```python
from build123d import *

# Parameters (mm, degrees)
SKETCH1_R                = 5
SKETCH1_R_2              = 4
BOSS_EXTRUDE1_DEPTH      = 5
BOSS_EXTRUDE3_DEPTH      = 7.5
BOSS_EXTRUDE3_DEPTH_BACK = 12.5
SKETCH2_R                = 7
SKETCH2_R_2              = 5
SKETCH3_R                = 5
BOSS_EXTRUDE4_DEPTH      = 5
FILLET1_R                = 4


with BuildPart() as part:
    # Sketch1 → Boss-Extrude1 (new body)
    with BuildSketch(Plane(origin=(0, 0, 0), x_dir=(0, 0, -1), z_dir=(1, 0, 0))):
        with BuildLine():
            Line((50, 221.0514346), (50, 161.0514346))
            ThreePointArc((50, 161.0514346), (26.21791649, 82.161607759), (20, 0))
            ThreePointArc((20, 0), (0, -20), (-20, 0))
            ThreePointArc((-20, 0), (-3.28398519, 116.315677296), (50, 221.0514346))
        make_face()
        Circle(SKETCH1_R, mode=Mode.SUBTRACT)
        with Locations((0, 47.625)):
            Circle(SKETCH1_R_2, mode=Mode.SUBTRACT)
        with Locations((1.573444046, 62.542247529)):
            Circle(SKETCH1_R_2, mode=Mode.SUBTRACT)
        with Locations((3.912796623, 77.358705591)):
            Circle(SKETCH1_R_2, mode=Mode.SUBTRACT)
        with Locations((7.013151247, 92.034801844)):
            Circle(SKETCH1_R_2, mode=Mode.SUBTRACT)
        with Locations((10.86160852, 106.532711232)):
            Circle(SKETCH1_R_2, mode=Mode.SUBTRACT)
        with Locations((15.437856468, 120.817596765)):
            Circle(SKETCH1_R_2, mode=Mode.SUBTRACT)
        with Locations((20.715135496, 134.858619736)):
            Circle(SKETCH1_R_2, mode=Mode.SUBTRACT)
        with Locations((26.661473463, 148.629642385)):
            Circle(SKETCH1_R_2, mode=Mode.SUBTRACT)
        with Locations((33.241055411, 162.109594216)):
            Circle(SKETCH1_R_2, mode=Mode.SUBTRACT)
        with Locations((-0.810748538, 32.646926465)):
            Circle(SKETCH1_R_2, mode=Mode.SUBTRACT)
    extrude(amount=BOSS_EXTRUDE1_DEPTH)

    # Sketch2 → Boss-Extrude3 (add, two sides: drawn at the far end of the back side and taken through both)
    with BuildSketch(Plane(origin=(5, 0, 0), x_dir=(0, 0, -1), z_dir=(1, 0, 0)).offset(-BOSS_EXTRUDE3_DEPTH_BACK)):
        Circle(SKETCH2_R)
        Circle(SKETCH2_R_2, mode=Mode.SUBTRACT)
    extrude(amount=BOSS_EXTRUDE3_DEPTH + BOSS_EXTRUDE3_DEPTH_BACK)

    # Sketch3 → Boss-Extrude4 (add)
    with BuildSketch(Plane(origin=(0, 0, -50), x_dir=(-1, 0, 0), z_dir=(0, 0, -1))):
        with BuildLine():
            Line((-12.5, 151.0514346), (7.5, 151.0514346))
            ThreePointArc((7.5, 151.0514346), (14.571067812, 153.980366789), (17.5, 161.0514346))
            Line((17.5, 161.0514346), (17.5, 221.0514346))
            ThreePointArc((17.5, 221.0514346), (14.571067812, 228.122502412), (7.5, 231.0514346))
            Line((7.5, 231.0514346), (-12.5, 231.0514346))
            ThreePointArc((-12.5, 231.0514346), (-19.571067812, 228.122502412), (-22.5, 221.0514346))
            Line((-22.5, 221.0514346), (-22.5, 161.0514346))
            ThreePointArc((-22.5, 161.0514346), (-19.571067812, 153.980366789), (-12.5, 151.0514346))
        make_face()
        with Locations((-13.75, 221.0514346)):
            Circle(SKETCH3_R, mode=Mode.SUBTRACT)
        with Locations((-13.75, 206.0514346)):
            Circle(SKETCH3_R, mode=Mode.SUBTRACT)
        with Locations((-13.75, 191.0514346)):
            Circle(SKETCH3_R, mode=Mode.SUBTRACT)
        with Locations(Location((-13.75, 161.0514346, 0), (0, 0, 180))):
            Circle(SKETCH3_R, mode=Mode.SUBTRACT)
        with Locations(Location((-13.75, 176.0514346, 0), (0, 0, 180))):
            Circle(SKETCH3_R, mode=Mode.SUBTRACT)
        with Locations((8.75, 161.0514346)):
            Circle(SKETCH3_R, mode=Mode.SUBTRACT)
        with Locations((8.75, 176.0514346)):
            Circle(SKETCH3_R, mode=Mode.SUBTRACT)
        with Locations(Location((8.75, 191.0514346, 0), (0, 0, 180))):
            Circle(SKETCH3_R, mode=Mode.SUBTRACT)
        with Locations(Location((8.75, 206.0514346, 0), (0, 0, 180))):
            Circle(SKETCH3_R, mode=Mode.SUBTRACT)
        with Locations(Location((8.75, 221.0514346, 0), (0, 0, 180))):
            Circle(SKETCH3_R, mode=Mode.SUBTRACT)
    extrude(amount=BOSS_EXTRUDE4_DEPTH)

    # Fillet1
    fillet1_edges = [part.edges().sort_by_distance(p)[0] for p in [
        (5, 0, 7),
        (0, 0, 7),
    ]]
    fillet(fillet1_edges, radius=FILLET1_R)


solid = part.part
```
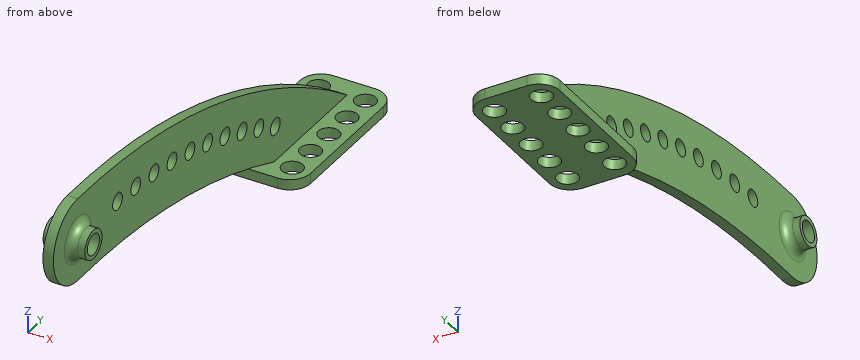
Source: CAD feature listing. Evaluate the final solid. Frame: model axes, mm. Give positions to 0.01 mm unless a question says otherwise; leave off trailing zeros. Loops run counter-clockwise (first coordinate to the right, second up) from the corner with the lowest first, then second, coordinate; pieces in that order, holes last. Notation, with made-up numbers: (82, -29.5) -> (138, -29.5) arc R31 cw to (138, 8.5) -> close; hole circle Ø5 at (30.5, 3). An arc over 180 degrees is marked (long way). Use a Markdown table: item, result. Add a question column.
(1) Section query B-B (y = 15). Output: boundary loops of the cut face in (x, z).
(2) Section query A-A (x = 16). Output: boundary loops of the cut face in (y, z), then the cut area to 3 significant figures.
(3) First-contact query: pin 1 Ø11.5 at (x, y) = (-8.75, 161.05) entering from +Z; pin 2 Ø5.5 at (x, z) = (6, -51.5) entering from -Y; pin 3 Ø2 at (y, z) = (114, 4) entering from -X. Flat tips, straight axial feed; report the tip coordinate or a pass-through.
(4) Ray query, line 1 (X direction, y = 9, z = -8); line 2 (Y direction, x = -8.75, z = -52.25); line 3 (Z direction, x = 10, y = 167). Return the intervals inside material, ascending.
Checked values:
| question | item | result |
|---|---|---|
| 1 | outline | (0, -19.8) -> (5, -19.8) -> (5, 20.01) -> (0, 20.01) -> close |
| 2 | outline | (151.68, -55) -> (156.59, -55) -> (156.59, -50) -> (151.68, -50) -> close; (165.52, -55) -> (171.59, -55) -> (171.59, -50) -> (165.52, -50) -> close; (180.52, -55) -> (186.59, -55) -> (186.59, -50) -> (180.52, -50) -> close; (195.52, -55) -> (201.59, -55) -> (201.59, -50) -> (195.52, -50) -> close; (210.52, -55) -> (216.59, -55) -> (216.59, -50) -> (210.52, -50) -> close; (225.52, -55) -> (230.42, -55) -> (230.42, -50) -> (225.52, -50) -> close |
| 2 | area | 170 mm^2 |
| 3 | pin 1 | z = -50 |
| 3 | pin 2 | y = 151.05 |
| 3 | pin 3 | x = 0 |
| 4 | line 1 | 0 to 5 |
| 4 | line 2 | 151.13 to 156.05, 166.05 to 171.05, 181.05 to 186.05, 196.05 to 201.05, 211.05 to 216.05, 226.05 to 230.97 |
| 4 | line 3 | -55 to -50 |
